from build123d import *

# Parameters (mm, degrees)
F1_DEPTH      = 254
F3_DEPTH      = 254
F3_DEPTH_BACK = 254
F4_R          = 12.7
F5_DEPTH      = 254


with BuildPart() as f1:
    # F0 (on Top) → F1 (new body)
    with BuildSketch(Plane.XY):
        with BuildLine():
            Line((-63.5, 0), (63.5, 0))
            ThreePointArc((63.5, 0), (0, 63.5), (-63.5, 0))
        make_face()
        with BuildLine():
            Line((63.5, -381), (63.5, 0))
            ThreePointArc((63.5, 0), (0, -63.5), (-63.5, 0))
            Line((-63.5, 0), (-63.5, -381))
            ThreePointArc((-63.5, -381), (0, -317.5), (63.5, -381))
        make_face()
        with BuildLine():
            ThreePointArc((-63.5, 0), (0, -63.5), (63.5, 0))
            Line((63.5, 0), (-63.5, 0))
        make_face()
        with BuildLine():
            ThreePointArc((-63.5, -381), (0, -444.5), (63.5, -381))
            Line((63.5, -381), (-63.5, -381))
        make_face()
        with BuildLine():
            Line((-63.5, -381), (63.5, -381))
            ThreePointArc((63.5, -381), (0, -317.5), (-63.5, -381))
        make_face()
    extrude(amount=F1_DEPTH)

    # F2 (on Right) → F3 (cut, two sides)
    with BuildSketch(Plane.YZ) as f3_sk:
        Polygon((-487.0654642582, 308.1015944481), (-487.0654642582, 101.9910350442), (-204.5872807503, 308.1015944481), align=None)
    extrude(amount=-F3_DEPTH, mode=Mode.SUBTRACT)
    extrude(f3_sk.sketch, amount=F3_DEPTH_BACK, mode=Mode.SUBTRACT)

    # F4 (on Top) → F5 (cut)
    with BuildSketch(Plane.XY):
        with Locations((0, -381)):
            Circle(F4_R)
    extrude(amount=F5_DEPTH, mode=Mode.SUBTRACT)


solid = f1.part
Here's how the part is built. I have some questions about the finished solid (model axes, mm). Coordinates: 2 decimals unless noted, no trailing zeros. Order: outer loops, then holes, each group sorted by start corner. A loop starts at its lowest first (then second) coordinate and runs counter-clockwise, first axis right, second up. Notation, with made-up numbers: (6.25, 34) -> (46.25, 34) arc R19 cw to (46.25, 56) -> close; hole circle Ø11 at (50.5, 27). An arc over 180 degrees is marked (long way). Answer in a Markdown table with one row per item.
(1) Thinking about a two-plate mould opening in X: for faces 1 (the face through (-1.653, -368.408, 93.004)), 2 (the face through (-63.5, -188, 125)), 3 (the face through (63.5, -193, 125)), 4 (the face through (-0.889, -362.778, 192.678)), which applies, +X half, -X half, draft (parallel to the pull), parting line (faces both ways), or undercut?
Answer key:
| item | result |
|---|---|
| face 1 | undercut |
| face 2 | -X half |
| face 3 | +X half |
| face 4 | draft |
(2) I want a section at D-D on z = 156.5. List the corners of the cut face in (x, y) for me.
Answer key:
| item | result |
|---|---|
| outline | (-63.5, -381) arc R63.5 ccw to (-55.22, -412.36) -> (55.22, -412.36) arc R63.5 ccw to (63.5, -381) -> (63.5, 0) arc R63.5 ccw to (-63.5, 0) -> close; hole circle Ø25.4 at (0, -381) |
(3) I want a section at A-A on x = 0. List the corners of the cut face in (y, z) for me, then the cut area to 3 significant figures.
Answer key:
| item | result |
|---|---|
| outline | (-444.5, 0) -> (-393.7, 0) -> (-393.7, 170.12) -> (-444.5, 133.05) -> close; (-368.3, 0) -> (63.5, 0) -> (63.5, 254) -> (-278.73, 254) -> (-368.3, 188.65) -> close |
| area | 114,000 mm^2 |
(4) Please list where these lines run through material, in increasing order: probe 1 along Y at (x, z) = (0, 93); probe 2 along X at (y, z) = (-381, 141); probe 3 along Y at (x, z) = (-0.5, 187).
Answer key:
| item | result |
|---|---|
| probe 1 | -444.5 to -393.7, -368.3 to 63.5 |
| probe 2 | -63.5 to -12.7, 12.7 to 63.5 |
| probe 3 | -368.31 to 63.5 |
(5) I want a section at B-B on z = 75. List the corners of the cut face in (x, y) for me, then the cut area to 3 significant figures.
Answer key:
| item | result |
|---|---|
| outline | (-63.5, -381) arc R63.5 ccw to (63.5, -381) -> (63.5, 0) arc R63.5 ccw to (-63.5, 0) -> close; hole circle Ø25.4 at (0, -381) |
| area | 60,500 mm^2 |
(6) Will these pins go through, and if not, where does the flat tip stop? pin 1 Ø4 at (x, z) = (-50, 149.5) entering from -Y; pin 2 Ø4 at (x, z) = (-22, 171.5) entering from +Y; pin 3 Ø2 at (x, y) = (20, -193.5) entering from -Z; pin 4 Ø10 at (x, z) = (-40, 137.5) entering from -Y.
Answer key:
| item | result |
|---|---|
| pin 1 | y = -422.52 |
| pin 2 | y = 60.27 |
| pin 3 | z = 0 |
| pin 4 | y = -433.98 |
(7) I want a section at C-C on x = 27. List the corners of the cut face in (y, z) for me.
Answer key:
| item | result |
|---|---|
| outline | (-438.47, 0) -> (57.47, 0) -> (57.47, 254) -> (-278.73, 254) -> (-438.47, 137.45) -> close |
